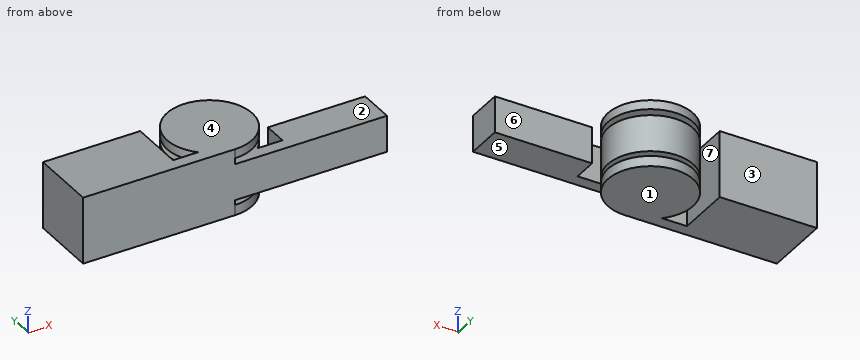
from build123d import *

# Parameters (mm, degrees)
BOSS_EXTRUDE1_DEPTH      = 139.7
SKETCH2_R                = 88.9
CUT_EXTRUDE1_DEPTH       = 50.8
CUT_EXTRUDE1_DEPTH_BACK  = 48.26
BOSS_EXTRUDE3_DEPTH      = 38.1
BOSS_EXTRUDE3_DEPTH_BACK = 38.1


with BuildPart() as part:
    # Sketch1 → Boss-Extrude1 (new body)
    with BuildSketch(Plane.XY):
        with BuildLine():
            Line((0, 0), (203.2, 0))
            Line((203.2, 0), (317.5, 0))
            ThreePointArc((317.5, 0), (351.101041651, 171.20540687), (255.282960533, 25.4))
            Line((255.282960533, 25.4), (203.2, 25.4))
            Line((203.2, 25.4), (203.2, 139.7))
            Line((203.2, 139.7), (0, 139.7))
            Line((0, 139.7), (0, 0))
        make_face()
    extrude(amount=BOSS_EXTRUDE1_DEPTH)

    # Sketch2 → Cut-Extrude1 (cut, two sides)
    with BuildSketch(Plane.XY.offset(69.85)) as cut_extrude1_sk:
        with Locations((317.5, 88.9)):
            Circle(SKETCH2_R)
    extrude(amount=CUT_EXTRUDE1_DEPTH, mode=Mode.SUBTRACT)
    extrude(cut_extrude1_sk.sketch, amount=-CUT_EXTRUDE1_DEPTH_BACK, mode=Mode.SUBTRACT)

    # Sketch5 → Boss-Extrude3 (add, two sides)
    with BuildSketch(Plane.XY.offset(69.85)) as boss_extrude3_sk:
        with BuildLine():
            Line((317.5, 0), (431.8, 0))
            Line((431.8, 0), (635, 0))
            Line((635, 0), (635, 76.2))
            Line((635, 76.2), (431.8, 76.2))
            Line((431.8, 76.2), (431.8, 25.4))
            Line((431.8, 25.4), (379.717039467, 25.4))
            ThreePointArc((379.717039467, 25.4), (283.898958349, 171.20540687), (317.5, 0))
        make_face()
    extrude(amount=BOSS_EXTRUDE3_DEPTH)
    extrude(boss_extrude3_sk.sketch, amount=-BOSS_EXTRUDE3_DEPTH_BACK)


solid = part.part
The listing builds one solid part. Answer for the finished solid, in the listing's coordinates (mm). Face numbers are marked on the shaded views. A direction names the side the tool comes from. Give positions to 0.01 mm unless a question says otherwise; leave off trailing zeros. Write each loop counter-clockwise with the first axis right and the second up, starting at its lowest first coordinate (ties: lowest second). Pieces come first, ordered by that corner, then holes. Notation, with made-up numbers: (21, 45.25) -> (76, 45.25) arc R18 ccw to (76, 65.25) -> close; hole circle Ø1 at (39, 79). An arc over 180 degrees is marked (long way). Use a Markdown table: item, result.
(1) Section C-C, the plane z = 75.5 is taken. Determine the outline of the cut face in (x, y).
Return value:
| item | result |
|---|---|
| outline | (0, 0) -> (635, 0) -> (635, 76.2) -> (431.8, 76.2) -> (431.8, 25.4) -> (379.72, 25.4) arc R88.9 ccw (long way) to (255.28, 25.4) -> (203.2, 25.4) -> (203.2, 139.7) -> (0, 139.7) -> close |
(2) Section D-D, the plane y = 154 is taken. Determine the outline of the cut face in (x, z).
Return value:
| item | result |
|---|---|
| outline | (256.96, 0) -> (378.04, 0) -> (378.04, 21.59) -> (256.96, 21.59) -> close; (256.96, 31.75) -> (378.04, 31.75) -> (378.04, 107.95) -> (256.96, 107.95) -> close; (256.96, 120.65) -> (378.04, 120.65) -> (378.04, 139.7) -> (256.96, 139.7) -> close |
(3) Flat-ended cylindrical pins translate along their axes: P1, Ø6, axis at x = 488, y = 55, coming from the +Z side; P2, Ø8, axis at y = 114, z = 16.5, coming from the +X side; P3, Ø8, axis at x = 510.5, z = 99, coming from the +Y side. Find the tip coordinate at first contact, or state that the pin passes through.
Return value:
| item | result |
|---|---|
| P1 | z = 107.95 |
| P2 | x = 403.86 |
| P3 | y = 76.2 |
(4) For the marked faces 4, 5, 6 and 7, determine the directions among +Z, -Z, +X, -X, +Y, -Y from which every point of the face is accessible in a straight line to the end or side of a thin tool.
Return value:
| item | result |
|---|---|
| face 4 | +Z, +X, -X, +Y, -Y |
| face 5 | +X, +Y |
| face 6 | +Z, -Z, +X, +Y |
| face 7 | +Z, -Z, +Y |
(5) Determine the mould class of the marked faces 1, 2 and 3 for opening direction Z: released by +Z, released by -Z, zero draft, split by the parting line, or undercut.
Return value:
| item | result |
|---|---|
| face 1 | released by -Z |
| face 2 | undercut |
| face 3 | zero draft |
(6) Section B-B, the plane x = 391 is taken. Determine the outline of the cut face in (y, z).
Return value:
| item | result |
|---|---|
| outline | (0, 31.75) -> (25.4, 31.75) -> (25.4, 107.95) -> (0, 107.95) -> close; (38.89, 0) -> (138.91, 0) -> (138.91, 21.59) -> (38.89, 21.59) -> close; (38.89, 31.75) -> (138.91, 31.75) -> (138.91, 107.95) -> (38.89, 107.95) -> close; (38.89, 120.65) -> (138.91, 120.65) -> (138.91, 139.7) -> (38.89, 139.7) -> close |
(7) Section A-A, the plane y = 88.9 is taken. Determine the outline of the cut face in (x, z), then the cut area to 3 significant figures.
Return value:
| item | result |
|---|---|
| outline | (0, 0) -> (203.2, 0) -> (203.2, 139.7) -> (0, 139.7) -> close; (228.6, 0) -> (406.4, 0) -> (406.4, 21.59) -> (228.6, 21.59) -> close; (228.6, 31.75) -> (406.4, 31.75) -> (406.4, 107.95) -> (228.6, 107.95) -> close; (228.6, 120.65) -> (406.4, 120.65) -> (406.4, 139.7) -> (228.6, 139.7) -> close |
| area | 49,200 mm2 |
(8) Find the intervals of material crossed by probe 1 along Z at (x, y) = (345, 34.5); probe 2 along X at (y, z) = (46, 83); probe 3 along X at (y, z) = (126.5, 58), in increasing order. Write a range as from..to.
Return value:
| item | result |
|---|---|
| probe 1 | 0..21.59, 31.75..107.95, 120.65..139.7 |
| probe 2 | 0..203.2, 239.64..395.36, 431.8..635 |
| probe 3 | 0..203.2, 236.94..398.06 |
